Geometry check sheet. Reference: the model listing, model coordinates, mm. A direction names the side the tool comes from. Round coordinates to 2 decimals unless told otherwise and drop trailing zeros. Order: outer loops, then holes, each group sorted by start corner. A loop starts at its lowest first (then second) coordinate and runs counter-clockwise, first axis right, second up. Notation, with made-up numbers: (25.25, 64.5) - (79.25, 64.5) arc R18 ccw to (79.25, 94.5) - close; hole circle Ø3 at (20, 8). An arc over 180 degrees is marked (long way). Use a Markdown table: item, result. Add a question column.
(1) Mould release check, pull along X, two halves, no side actions. Record for faces 3 (the face through (187.325, -1, 9)), 4 (the face through (-114.3, -1, 9)), 5 (the face through (4, 1, 19.05)), 6 (the face through (-30, 1, 12.7)): released by +X, released by -X, zero draft, split by the parting line, or undercut.
(2) Gauge pin test, flat ends, axial feed: P1, Ø5.5, axis at x = 17.46, y = 0, coming from the -Z side; P2, Ø1.9, axis at y = 28.97, z = 9.52, coming from the -X side; P3, Ø5, axis at x = -30.5, y = 6.5, coming from the +Z side. Record the tip position at first contact, or that the pin passes through.
(3) Thickness scan on line 1 along X through (y, z) = (-34.5, 15) (1 decimal); line 2 along Z through (x, y) = (-32.5, -32.5). Record the ranges inside material, lowest first. Write a range as [from, to].
(4) Access from +Z, -Z, +X, -X, +Y, -Y to the whole of each face (thin tool, end or side, straight path). Record for faces 1 (the face through (34, -41.275, 9)), 2 (the face through (36.512, -1, 16)).
(5) Section check A-A on z = 15.25. Record the boundary of the cut face in (x, y) (1 decimal), then the cut area to 3 significant figures.
```python
from build123d import *

# Parameters (mm, degrees)
F0_W           = 301.625
F0_H           = 82.55
F1_DEPTH       = 19.05
F2_W           = 6.35
F2_H           = 82.55
F3_DEPTH       = 6.35
F5_D           = 4.572
F5_CSINK_D     = 9.1186
F5_CSINK_ANGLE = 82
F7_D           = 3.175
F7_DEPTH       = 12.7
F7_TIP         = 0.9538662327


with BuildPart() as f1:
    # F0 (on Top) → F1 (new body)
    with BuildSketch(Plane.XY):
        with Locations((36.5125, 0)):
            Rectangle(F0_W, F0_H)
    extrude(amount=F1_DEPTH)

    # F2 (on face) → F3 (cut)
    with BuildSketch(Plane.XY.offset(19.05)):
        with Locations((-30.1625, 0)):
            Rectangle(F2_W, F2_H)
        with Locations((39.6875, 0)):
            Rectangle(F2_W, F2_H)
    extrude(amount=-F3_DEPTH, mode=Mode.SUBTRACT)

    # F5 (through all)
    with Locations(Plane(origin=(0, 0, 0), x_dir=(1, 0, 0), z_dir=(0, 0, -1))):
        with Locations((17.4625, 0)):
            CounterSinkHole(F5_D / 2, F5_CSINK_D / 2, counter_sink_angle=F5_CSINK_ANGLE)

    # F7
    with Locations(Plane(origin=(-114.3, 0, 0), x_dir=(0, -1, 0), z_dir=(-1, 0, 0))):
        with Locations((-28.9729410976, 9.525), (28.1770589024, 9.525)):
            Hole(F7_D / 2, depth=F7_DEPTH)
            with Locations((0, 0, -(F7_DEPTH + F7_TIP / 2))):  # 118° drill point
                Cone(0, F7_D / 2, F7_TIP, mode=Mode.SUBTRACT)


solid = f1.part
```
Check sheet entries:
| question | item | result |
|---|---|---|
| 1 | face 3 | released by +X |
| 1 | face 4 | released by -X |
| 1 | face 5 | zero draft |
| 1 | face 6 | undercut |
| 2 | P1 | stops at z = 2.08 |
| 2 | P2 | stops at x = -101.22 |
| 2 | P3 | stops at z = 12.7 |
| 3 | line 1 | x = [-114.3, -33.3], [-27, 36.5], [42.9, 187.3] |
| 3 | line 2 | z = [0, 12.7] |
| 4 | face 1 | +Z, -Z, +X, -X, -Y |
| 4 | face 2 | +Z, +Y, -Y |
| 5 | outline | (-114.3, -41.3) - (-33.3, -41.3) - (-33.3, 41.3) - (-114.3, 41.3) - close; (-27, -41.3) - (36.5, -41.3) - (36.5, 41.3) - (-27, 41.3) - close; (42.9, -41.3) - (187.3, -41.3) - (187.3, 41.3) - (42.9, 41.3) - close; hole circle Ø4.6 at (17.5, 0) |
| 5 | area | 23,800 mm2 |
